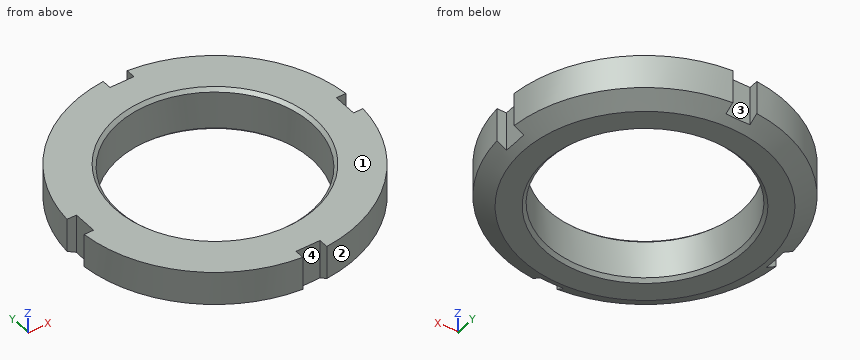
Autodesk Inventor part; units mm, degrees
ref_plane "wash_to_nut_XY" through (0, 0, -11) normal (0, 0, 1) x (1, 0, 0)
ref_plane "wash_to_nut_YZ" through (0, 0, -11) normal (1, 0, 0) x (0, 1, 0)
ref_plane "wash_to_nut_ZX" through (0, 0, -11) normal (0, 1, 0) x (0, 0, 1)
sketch "Sketch_1" plane through (0, 0, 0) normal (1, 0, 0) x (0, 1, 0)
  line L0 (0, -11) -> (0, 0)
  line L1 (25, 0) -> (24.188, -0.812)
  line L2 (24.188, -0.812) -> (24.188, -10.188)
  line L3 (24.188, -10.188) -> (25, -11)
  line L4 (25, -11) -> (30.5, -11)
  line L5 (30.5, -11) -> (35, -8.4019)
  line L6 (35, -8.4019) -> (35, 0)
  line L7 (35, 0) -> (25, 0)
revolve "Revolution1" add sketch "Sketch_1" angle 360 about axis through (0, 0, -11) along (0, 0, -1)
thread "Thread1"
sketch "Sketch_2" plane through (0, 0, 0) normal (0, 0, 1) x (1, 0, 0)
  circle A0 centre (0, 0) radius 70
  arc A1 (-53.7625, -3) -> (-3, -53.7625) centre (0, 0) ccw
  line L0 (-3, -53.7625) -> (-3, -32.5)
  line L1 (-3, -32.5) -> (3, -32.5)
  line L2 (3, -32.5) -> (3, -53.7625)
  arc A2 (3, -53.7625) -> (53.7625, -3) centre (0, 0) ccw
  line L3 (53.7625, -3) -> (32.5, -3)
  line L4 (32.5, -3) -> (32.5, 3)
  line L5 (32.5, 3) -> (53.7625, 3)
  arc A3 (53.7625, 3) -> (3, 53.7625) centre (0, 0) ccw
  line L6 (3, 53.7625) -> (3, 32.5)
  line L7 (3, 32.5) -> (-3, 32.5)
  line L8 (-3, 32.5) -> (-3, 53.7625)
  arc A4 (-3, 53.7625) -> (-53.7625, 3) centre (0, 0) ccw
  line L9 (-53.7625, 3) -> (-32.5, 3)
  line L10 (-32.5, 3) -> (-32.5, -3)
  line L11 (-32.5, -3) -> (-53.7625, -3)
extrude "Extrusion1" cut sketch "Sketch_2" against normal blind 11
ref_plane "wash_to_nut_XY" through (0, 0, -11) normal (0, 0, 1) x (1, 0, 0)
ref_plane "wash_to_nut_YZ" through (0, 0, -11) normal (1, 0, 0) x (0, 1, 0)
ref_plane "wash_to_nut_ZX" through (0, 0, -11) normal (0, 1, 0) x (0, 0, 1)
properties part number "JLNSK50nut"
Could you check a few things on this model? Use its own coordinates, in mm. Face numbers are marked on the shaded views. Coordinates: 2 decimals unless noted, no trailing zeros. Loops run counter-clockwise (first coordinate to the right, second up) from the corner with the lowest first, then second, coordinate; pieces in that order, holes last. Notation, with made-up numbers: M -38.75,-36.5 L -25.75,-36.5 A13 ccw -25.75,-28.5 Z; hole C 35.25,39 d8. An arc over 180 degrees is marked long. Put each result on its own line as item: value. Start each with the question number.
(1) Suppose I cut it at A-A on x = 0. Please give me the cut outline in (y, z), then the cut area to 3 significant figures.
(2) I need wall thicknesses on line 1 (X direction, y = 0, z = -7.5); line 2 (Y direction, x = -17, z = -3); line 3 (Y direction, x = -15.5, z = -1.25). Which ranges of each line are inside material? Lowest first, please. Write a range as from..to.
(3) Thinking about a two-plate mould opening in X: for the marked faces 1, 2, 3 and 4, which applies, pulls with the +X half, pulls with the -X half, needs draft (parallel to the pull), parting line crosses it, or undercut?
(4) Will these pins go through, and if not, where does the flat tip stop? P1, Ø1.8, axis at y = -1, z = -6, coming from the -X side; P2, Ø3, axis at y = -12, z = -7, coming from the +X side; P3, Ø1.2, axis at y = -33, z = -5, coming from the -X side.
(5) Suppose I cut it at C-C on z = -2.75. Please give me the cut outline in (x, y).
Solutions:
1. outline: M -32.5,-9.85 L -30.5,-11 L -25,-11 L -24.19,-10.19 L -24.19,-0.81 L -25,0 L -32.5,0 Z; M 24.19,-10.19 L 25,-11 L 30.5,-11 L 32.5,-9.85 L 32.5,0 L 25,0 L 24.19,-0.81 Z
1. area: 179 mm2
2. line 1: x = -32.5..-24.19, 24.19..32.5
2. line 2: y = -30.59..-17.21, 17.21..30.59
2. line 3: y = -31.38..-18.57, 18.57..31.38
3. face 1: needs draft
3. face 2: pulls with the +X half
3. face 3: undercut
3. face 4: undercut
4. P1: stops at x = -32.5
4. P2: stops at x = 33.39
4. P3: stops at x = -13.24
5. outline: M -34.87,-3 A35 ccw -3,-34.87 L -3,-32.5 L 3,-32.5 L 3,-34.87 A35 ccw 34.87,-3 L 32.5,-3 L 32.5,3 L 34.87,3 A35 ccw 3,34.87 L 3,32.5 L -3,32.5 L -3,34.87 A35 ccw -34.87,3 L -32.5,3 L -32.5,-3 Z; hole C 0,0 d48.38
